```python
from build123d import *

# Parameters (mm, degrees)
REVOLVE1_ANGLE                                      = 110
BOSS_EXTRUDE2_START                                 = 2
BOSS_EXTRUDE2_DEPTH                                 = 2
CUT_EXTRUDE3_DEPTH                                  = 4.3
CUT_EXTRUDE3_DEPTH_BACK                             = 4.3
SKETCH6_W                                           = 4.978949903
SKETCH6_H                                           = 35.147852634
CSK_FOR_M3_COUNTERSUNK_FLAT_HEAD_SCREW1_D           = 3.4
CSK_FOR_M3_COUNTERSUNK_FLAT_HEAD_SCREW1_CSINK_D     = 6.3
CSK_FOR_M3_COUNTERSUNK_FLAT_HEAD_SCREW1_CSINK_ANGLE = 90
CUT_EXTRUDE4_DEPTH                                  = 58.131427582
CUT_EXTRUDE5_DEPTH                                  = 4


with BuildPart() as part:
    # Sketch1 → Revolve1 (revolve)
    with BuildSketch(Plane.XY):
        Polygon((-29, 0), (-29, 8), (-40, 8), (-39.896417966, 0.000670605), align=None)
    revolve(axis=Axis((0, 0, 0), (0, 1, 0)), revolution_arc=REVOLVE1_ANGLE)

    # Sketch2 → Boss-Extrude2 (add)
    with BuildSketch(Plane(origin=(0, 8, 0), x_dir=(1, 0, 0), z_dir=(0, 1, 0)).offset(BOSS_EXTRUDE2_START)):
        with BuildLine():
            Line((-29, 0), (-30.5, 0))
            ThreePointArc((-30.5, 0), (-17.494081309, -24.984137351), (10.431614371, -28.660624934))
            Line((10.431614371, -28.660624934), (9.918584156, -27.251086003))
            ThreePointArc((9.918584156, -27.251086003), (-16.633716654, -23.755409284), (-29, 0))
        make_face()
    extrude(amount=-BOSS_EXTRUDE2_DEPTH)

    # Sketch6 → Cut-Extrude3 (cut, two sides: drawn at the far end of the back side and taken through both)
    with BuildSketch(Plane(origin=(0, 0, 0), x_dir=(0.5735764363510444, 0, -0.819152044288993), z_dir=(0.819152044288993, 0, 0.5735764363510444)).offset(-CUT_EXTRUDE3_DEPTH_BACK)):
        with Locations((-37.788406982, 11.886060953)):
            Rectangle(SKETCH6_W, SKETCH6_H)
    extrude(amount=CUT_EXTRUDE3_DEPTH + CUT_EXTRUDE3_DEPTH_BACK, mode=Mode.SUBTRACT)

    # CSK for M3 Countersunk Flat Head Screw1 (through all)
    with Locations(Plane(origin=(-16.693228701, 3.799474552, 23.713627212), x_dir=(-0.817711283166, 0, -0.575628575891), z_dir=(0.575628575891, 0, -0.817711283166))):
        with Locations((0, 0)):
            CounterSinkHole(CSK_FOR_M3_COUNTERSUNK_FLAT_HEAD_SCREW1_D / 2, CSK_FOR_M3_COUNTERSUNK_FLAT_HEAD_SCREW1_CSINK_D / 2, counter_sink_angle=CSK_FOR_M3_COUNTERSUNK_FLAT_HEAD_SCREW1_CSINK_ANGLE)

    # Sketch13 → Cut-Extrude4 (cut, through all)
    with BuildSketch(Plane(origin=(0, 8, 0), x_dir=(1, 0, 0), z_dir=(0, 1, 0))):
        Polygon((-23.768989432, -26.448813658), (-29.09347772, -22.720566822), (-32.344693082, -27.363783561), (-27.020204794, -31.092030397), align=None)
    extrude(amount=-CUT_EXTRUDE4_DEPTH, mode=Mode.SUBTRACT)

    # Sketch14 → Cut-Extrude5 (cut)
    with BuildSketch(Plane(origin=(0, 8, 0), x_dir=(1, 0, 0), z_dir=(0, 1, 0))):
        Polygon((-29.09347772, -22.720566822), (-23.756197421, -26.457770721), (-22.0628619, -24.039436971), (-27.202235941, -20.019593646), align=None)
    extrude(amount=-CUT_EXTRUDE5_DEPTH, mode=Mode.SUBTRACT)


solid = part.part
```
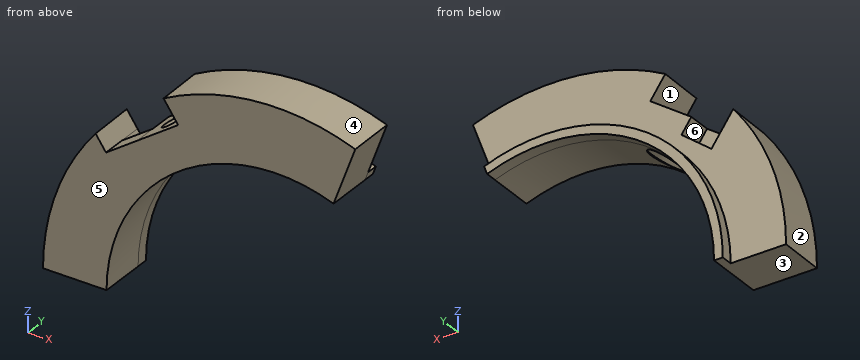
Geometry: final body of the model. Coordinates: model frame, mm. Face numbers are marked on the shaded views. A direction names the side the tool comes from. Coordinates: 2 decimals unless noted, no trailing zeros. Return JSON: item names as keys, results as strings. Group by question number.
1. Pin query (flat end, axial travel): pin 1 (1.5 mm diameter, centred on y = 3, z = 18.5, fed in from -X); pin 2 (6 mm diameter, centred on x = -22.5, y = 8, fed in from -Z); pin 3 (1.5 mm diameter, centred on y = 9, z = 18, fed in from -X). Return the tip coordinate at first contact, or that it passes through.
2. Pull-direction query (X, two-part tool) for the marked faces 4, 5 and 6; classes: pulls with the +X half, pulls with the -X half, needs draft (parallel to the pull), parting line crosses it, or undercut.
3. Material intervals for line 1 along Y through (x, z) = (-31.5, 8); line 2 along Z through (x, y) = (-23, 4.5); line 3 along Z through (x, y) = (-33.5, 1.5), sorted ascending. Write a range as [from, to].
4. Set-up query: the marked faces 1, 2 and 3. Return all of +Z, -Z, +X, -X, +Y, -Y with unobstructed straight access to the full face (end or side cutting, diameter ignored); none if empty.
Resolved:
{
 "1": {"pin 1": "stops at x = -35.77", "pin 2": "stops at z = 13.81", "pin 3": "stops at x = -25.15"},
 "2": {"face 4": "parting line crosses it", "face 5": "needs draft", "face 6": "undercut"},
 "3": {"line 1": "y = [0, 8]", "line 2": "z = [17.66, 23.31], [25.38, 26.99]", "line 3": "z = [0, 21.7]"},
 "4": {"face 1": "-X, +Y, -Y", "face 2": "+Z, -X, -Y", "face 3": "-Z, +X, -X, +Y, -Y"}
}
